from build123d import *

# Parameters (mm, degrees)
F1_DEPTH = 60
F2_SIZE  = 10
F3_R     = 2
F4_DEPTH = 25


with BuildPart() as f1:
    # F0 (on Top) → F1 (new body)
    with BuildSketch(Plane.XY):
        Polygon((0, 20), (0, 0), (41, 0), (41, 20), (38, 20), (38, 3), (3, 3), (3, 20), align=None)
    extrude(amount=F1_DEPTH)

    # F2
    f2_edges = [f1.edges().sort_by_distance(p)[0] for p in [
        (39.5, 20, 0),
        (1.5, 20, 0),
    ]]
    chamfer(f2_edges, length=F2_SIZE)

    # F3 (on face) → F4 (cut)
    with BuildSketch(Plane(origin=(0, 3, 0), x_dir=(-1, 0, 0), z_dir=(0, 1, 0))):
        with Locations((-14.5, 10)):
            Circle(F3_R)
        with Locations((-26.5, 10)):
            Circle(F3_R)
    extrude(amount=-F4_DEPTH, mode=Mode.SUBTRACT)


solid = f1.part
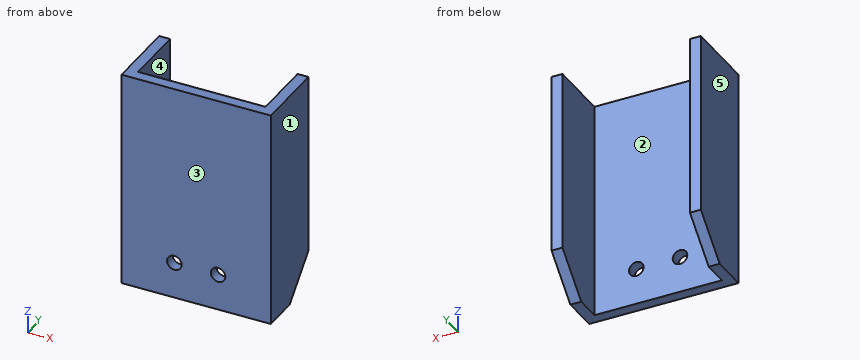
Source: CAD feature listing. Evaluate the final solid. Frame: model axes, mm. Face numbers are marked on the shaded views. A direction names the side the tool comes from. Give positions to 0.01 mm unless a question says otherwise; leave off trailing zeros. Write each loop counter-clockwise with the first axis right and the second up, starting at its lowest first coordinate (ties: lowest second). Pieces come first, ordered by that corner, then holes. Notation, with made-up numbers: M -29.75,17 L 12.25,17 A30 cw 12.25,53 Z; hole C 44.5,3.5 d9. An arc over 180 degrees is marked long. Return JSON: item names as keys, results as strings. Group by question number.
1) Pin query (flat end, axial travel): P1, Ø8, axis at x = 7, z = 13, coming from the -Y side; P2, Ø10, axis at x = 19.5, y = 11.5, coming from the -Z side; P3, Ø5, axis at x = 21.5, z = 20.5, coming from the +Y side. Return the tip coordinate at first contact, or that it passes through.
2) Pull-direction query (X, two-part tool) for the marked faces 3, 4 and 5; classes: pulls with the +X half, pulls with the -X half, needs draft (parallel to the pull), parting line crosses it, or undercut.
3) Material intervals for line 1 along Z through (x, y) = (26.5, 2.15); line 2 along X through (y, z) = (6.75, 43); line 3 along Y through (x, z) = (35, 42.5), sorted ascending. Write a range as [from, to].
4) Cut plane A-A, the plane x = 14.5. Output: boundary loops of the cut face in (y, z).
5) Cut plane D-D, the plane x = 32.5. Output: boundary loops of the cut face in (y, z), plus the area to 3 significant figures.
6) Set-up query: the marked faces 1 and 2. Return all of +Z, -Z, +X, -X, +Y, -Y with unobstructed straight access to the full face (end or side cutting, diameter ignored); none if empty.
7) Cut plane B-B, the plane y = 4.5. Output: boundary loops of the cut face in (x, z).
8) Cut plane C-C, the plane z = 15.5. Output: boundary loops of the cut face in (x, y), plus the area to 3 significant figures.
Recorded:
{
 "1": {"P1": "stops at y = 0", "P2": "passes through", "P3": "stops at y = 3"},
 "2": {"face 3": "needs draft", "face 4": "undercut", "face 5": "pulls with the -X half"},
 "3": {"line 1": "z = [0, 8], [12, 60]", "line 2": "x = [0, 3], [38, 41]", "line 3": "y = [0, 3]"},
 "4": {"outline": "M 0,0 L 3,0 L 3,8 L 0,8 Z; M 0,12 L 3,12 L 3,60 L 0,60 Z"},
 "5": {"outline": "M 0,0 L 3,0 L 3,60 L 0,60 Z", "area": "180 mm²"},
 "6": {"face 1": "+Z, -Z, +X, +Y, -Y", "face 2": "+Z, -Z, +Y"},
 "7": {"outline": "M 0,0 L 3,0 L 3,60 L 0,60 Z; M 38,0 L 41,0 L 41,60 L 38,60 Z"},
 "8": {"outline": "M 0,0 L 41,0 L 41,20 L 38,20 L 38,3 L 3,3 L 3,20 L 0,20 Z", "area": "225 mm²"}
}
